Build history of the part. All positions in model axes, mm. A direction names the side the tool comes from. Give positions to 0.01 mm unless a question says otherwise; leave off trailing zeros. Order: outer loops, then holes, each group sorted by start corner. A loop starts at its lowest first (then second) coordinate and runs counter-clockwise, first axis right, second up. Notation, with made-up numbers: (-15, -5) - (43, -5) arc R22 cw to (43, 15) - close; hole circle Ø7 at (-32.5, -22). An arc over 180 degrees is marked (long way). Use a Markdown table: item, result.
from build123d import *

# Parameters (mm, degrees)
BOSS_EXTRUDE1_DEPTH = 32
FILLET1_R           = 16
FILLET2_R           = 16
SKETCH2_R           = 10
BOSS_EXTRUDE2_DEPTH = 5


with BuildPart() as part:
    # Sketch1 → Boss-Extrude1 (new body)
    with BuildSketch(Plane.XY):
        Polygon((0, 0), (0, 54.4), (-5.201179862, 62.028885271), (-56.801179862, 62.028885271), (-64.430065133, 54.4), (-64.430065133, 0), (-66.630065133, 0), (-66.630065133, 54.4), (-56.801179862, 64.228885271), (-5.201179862, 64.228885271), (2.2, 54.4), (2.2, 0.000275755), align=None)
    extrude(amount=BOSS_EXTRUDE1_DEPTH)

    # Fillet1
    fillet1_edges = [part.edges().sort_by_distance(p)[0] for p in [
        (-65.530065133, 0, 0),
        (-65.530065133, 0, 32),
    ]]
    fillet(fillet1_edges, radius=FILLET1_R - 0.0001)  # a hair under: the kernel refuses the full size

    # Fillet2
    fillet2_edges = [part.edges().sort_by_distance(p)[0] for p in [
        (1.1, 0.000137878, 32),
        (1.1, 0.000137878, 0),
    ]]
    fillet(fillet2_edges, radius=FILLET2_R - 0.0001)  # a hair under: the kernel refuses the full size

    # Sketch2 → Boss-Extrude2 (add)
    with BuildSketch(Plane(origin=(-64.430065133, 0, 0), x_dir=(0, 0, -1), z_dir=(1, 0, 0))):
        with Locations(Location((-16, 16, 0), (0, 0, 180))):
            Circle(SKETCH2_R)
    boss_extrude2 = extrude(amount=BOSS_EXTRUDE2_DEPTH)

    # Mirror1: Boss-Extrude2 across plane
    add(boss_extrude2.mirror(Plane(origin=(-32.215032567, 0, 0), x_dir=(0, 0, 1), z_dir=(1, 0, 0))))


solid = part.part
1) Slice it at A-A (y = 36.5). Write the cut outline in (x, z).
Computed:
| item | result |
|---|---|
| outline | (-66.63, 0) - (-64.43, 0) - (-64.43, 32) - (-66.63, 32) - close; (0, 0) - (2.2, 0) - (2.2, 32) - (0, 32) - close |
2) Tool access for faces 1 (the flat face through (-60.56, 58.27, 15.78)), 2 (the cylindrical face through (-61.97, 13, 25.54)), 3 (the flat face through (-59.43, 16, 16)), 4 (the flat face through (-31, 64.229, 16)): list every direction of +Z, -Z, +X, -X, +Y, -Y with a clear straight run to the whole face (end or side of a thin tool).
Computed:
| item | result |
|---|---|
| face 1 | +Z, -Z |
| face 2 | none |
| face 3 | +Z, -Z, -Y |
| face 4 | +Z, -Z, +X, -X, +Y |
3) Wall check: line 1 (X direction, y = 51, z = 30); line 2 (Y direction, x = -36, z = 24.5); line 3 (X direction, y = 56.5, z = 6). Give the ranges that are in metal, low to high. Write a range as from..to.
Computed:
| item | result |
|---|---|
| line 1 | x = -66.63..-64.43, 0..2.2 |
| line 2 | y = 62.03..64.23 |
| line 3 | x = -64.53..-62.33, -1.43..0.62 |
4) Slice it at B-B (x = -61.5). Write the cut outline in (y, z), and give its area (3 significant figures).
Computed:
| item | result |
|---|---|
| outline | circle Ø20 at (16, 16); (57.33, 0) - (59.53, 0) - (59.53, 32) - (57.33, 32) - close |
| area | 385 mm² |
5) Slice it at D-D (x = -18). Write the cut outline in (y, z), and give its area (3 significant figures).
Computed:
| item | result |
|---|---|
| outline | (62.03, 0) - (64.23, 0) - (64.23, 32) - (62.03, 32) - close |
| area | 70.4 mm² |
6) Slice it at C-C (z = 9.5). Write the cut outline in (x, y), and give its area (3 significant figures).
Computed:
| item | result |
|---|---|
| outline | (-66.63, 1.38) - (-64.43, 1.38) - (-64.43, 8.4) - (-59.43, 8.4) - (-59.43, 23.6) - (-64.43, 23.6) - (-64.43, 54.4) - (-56.8, 62.03) - (-5.2, 62.03) - (0, 54.4) - (0, 23.6) - (-5, 23.6) - (-5, 8.4) - (0, 8.4) - (0, 1.38) - (2.2, 1.38) - (2.2, 54.4) - (-5.2, 64.23) - (-56.8, 64.23) - (-66.63, 54.4) - close |
| area | 535 mm² |
7) Two-plate mould, pull along Y, no slides. Class faces 5 (the flat face through (2.2, 28, 16)), 6 (the cylindrical face through (-65.545, 4.563, 27.189)), 7 (the cylindrical face through (-2.47, 13, 25.54)): +Y half, -Y half, draft (parallel to the pull), parting line (faces both ways), or undercut.
Computed:
| item | result |
|---|---|
| face 5 | draft |
| face 6 | -Y half |
| face 7 | undercut |
8) Pin check, flat tip, straight feed: P1, Ø8, axis at x = -42.5, z = 9.5, coming from the -Y side. Stop position of the tip, or through.
Computed:
| item | result |
|---|---|
| P1 | stops at y = 62.03 |
